Geometry check sheet. Reference: the model listing, model coordinates, mm. A direction names the side the tool comes from. Coordinates: 2 decimals unless noted, no trailing zeros. Write each loop counter-clockwise with the first axis right and the second up, starting at its lowest first coordinate (ties: lowest second). Pieces come first, ordered by that corner, then holes. Notation, with made-up numbers: M 71.5,45.5 L 99.5,45.5 A11 ccw 99.5,55.5 Z; hole C -3,29 d8. An arc over 180 degrees is marked long. Write item = value, one per line. Start each with the question number.
```python
from build123d import *

# Parameters (mm, degrees)
SKETCH3_R           = 10.16
BOSS_EXTRUDE1_DEPTH = 1.27
SKETCH4_R           = 1.905
BOSS_EXTRUDE2_DEPTH = 6.35
LPATTERN1_COUNT     = 4
LPATTERN1_PITCH     = 5.08
SKETCH6_R           = 0.889
CUT_EXTRUDE1_DEPTH  = 6.35
SKETCH7_R           = 0.9525
CUT_EXTRUDE2_DEPTH  = 6.35
SKETCH8_R           = 1.016
CUT_EXTRUDE3_DEPTH  = 6.35
SKETCH9_R           = 1.0795
CUT_EXTRUDE4_DEPTH  = 6.35


with BuildPart() as part:
    # Sketch3 → Boss-Extrude1 (new body)
    with BuildSketch(Plane(origin=(0, 0, 0), x_dir=(1, 0, 0), z_dir=(0, 1, 0))):
        with Locations(Location((0, 0, 0), (0, 0, 270))):
            Circle(SKETCH3_R)
    extrude(amount=BOSS_EXTRUDE1_DEPTH)

    # Sketch4 → Boss-Extrude2 (add)
    with BuildSketch(Plane(origin=(0, 1.27, 0), x_dir=(1, 0, 0), z_dir=(0, 1, 0))):
        with Locations(Location((-5.08, -5.08, 0), (0, 0, 270))):
            Circle(SKETCH4_R)
    boss_extrude2 = extrude(amount=BOSS_EXTRUDE2_DEPTH)

    # LPattern1: Boss-Extrude2 ×4
    with Locations(*[Vector(0.7071067811865476, 0, -0.7071067811865476) * (i * LPATTERN1_PITCH) for i in range(1, LPATTERN1_COUNT)]):
        add(boss_extrude2)

    # Sketch6 → Cut-Extrude1 (cut)
    with BuildSketch(Plane(origin=(0, 7.62, 0), x_dir=(1, 0, 0), z_dir=(0, 1, 0))):
        with Locations(Location((-5.08, -5.08, 0), (0, 0, 270))):
            Circle(SKETCH6_R)
    extrude(amount=-CUT_EXTRUDE1_DEPTH, mode=Mode.SUBTRACT)

    # Sketch7 → Cut-Extrude2 (cut)
    with BuildSketch(Plane(origin=(0, 7.62, 0), x_dir=(1, 0, 0), z_dir=(0, 1, 0))):
        with Locations(Location((-1.487897552, -1.487897552, 0), (0, 0, 270))):
            Circle(SKETCH7_R)
    extrude(amount=-CUT_EXTRUDE2_DEPTH, mode=Mode.SUBTRACT)

    # Sketch8 → Cut-Extrude3 (cut)
    with BuildSketch(Plane(origin=(0, 7.62, 0), x_dir=(1, 0, 0), z_dir=(0, 1, 0))):
        with Locations(Location((2.104204897, 2.104204897, 0), (0, 0, 270))):
            Circle(SKETCH8_R)
    extrude(amount=-CUT_EXTRUDE3_DEPTH, mode=Mode.SUBTRACT)

    # Sketch9 → Cut-Extrude4 (cut)
    with BuildSketch(Plane(origin=(0, 7.62, 0), x_dir=(1, 0, 0), z_dir=(0, 1, 0))):
        with Locations(Location((5.696307345, 5.696307345, 0), (0, 0, 270))):
            Circle(SKETCH9_R)
    extrude(amount=-CUT_EXTRUDE4_DEPTH, mode=Mode.SUBTRACT)


solid = part.part
```
Q1. Cross-section at C-C on z = 5.08. Enter the section's corners in (x, y) (3 decimals), and give its area (3 significant figures).
Q2. Cross-section at B-B on x = 6. Enter the section's corners in (y, z), and give its area (3 significant figures).
Q3. Draft check along X on faces 1 (the face through (10.074, 0.626, -1.323)), 2 (the face through (-2.3, 7.62, 2.3)), 3 (the face through (4.642, 4.489, -5.93)). Enter one of: pulls with the +X half, pulls with the -X half, needs draft (parallel to the pull), parting line crosses it, or undercut.
Q4. Gauge pin test, flat ends, axial feed: pin 1 (1 mm diameter, centred on x = -1.5, z = 1, fed in from +Y); pin 2 (1.1 mm diameter, centred on x = 5.5, z = -6, fed in from +Y). Record the tip position at first contact, or that the pin passes through.
Q5. Set-up check for faces 4 (the face through (0, 1.27, 0)), 5 (the face through (-5, 7.62, 4)): record each of +Z, -Z, +X, -X, +Y, -Y from which the full face is reachable in a straight line by a thin tool's end or side.
Q6. Cross-section at A-A on y = 5.75. Enter the section's corners in (x, z) (1 decimal).
Q7. Scan lines: L1, parallel to X at y = 4.5, z = 5.08 (3 decimals); L2, parallel to Y at x = -6, z = -4.5; L3, parallel to Z at x = 1.25, y = 4.75. Record each from-to range of solid material in increasing order.
Q8. Cross-section at D-D on y = 0.75. Enter the section's corners in (x, z).
Values found:
q1.outline = M -8.799,0 L 8.799,0 L 8.799,1.27 L -3.175,1.27 L -3.175,7.62 L -4.191,7.62 L -4.191,1.27 L -5.969,1.27 L -5.969,7.62 L -6.985,7.62 L -6.985,1.27 L -8.799,1.27 Z
q1.area = 35.3 mm²
q2.outline = M 0,-8.2 L 1.27,-8.2 L 1.27,-7.58 L 7.62,-7.58 L 7.62,-6.73 L 1.27,-6.73 L 1.27,-4.66 L 7.62,-4.66 L 7.62,-3.82 L 1.27,-3.82 L 1.27,8.2 L 0,8.2 Z
q2.area = 31.6 mm²
q3.face_1 = parting line crosses it
q3.face_2 = needs draft
q3.face_3 = undercut
q4.pin_1 = 7.62
q4.pin_2 = 1.27
q5.face_4 = +Y
q5.face_5 = +Z, -Z, +X, -X, +Y
q6.outline = C -5.1,5.1 d3.8; C -1.5,1.5 d3.8; C 2.1,-2.1 d3.8; C 5.7,-5.7 d3.8; hole C -5.1,5.1 d1.8; hole C -1.5,1.5 d1.9; hole C 2.1,-2.1 d2; hole C 5.7,-5.7 d2.2
q7.L1 = -6.985 to -5.969, -4.191 to -3.175
q7.L2 = 0 to 1.27
q7.L3 = -3.81 to -2.65, -1.55 to -0.4
q8.outline = C 0,0 d20.32
